Design review of the part built by this model. Coordinates are the model's own, in mm. A direction names the side the tool comes from. Give positions to 0.01 mm unless a question says otherwise; leave off trailing zeros. Loops run counter-clockwise (first coordinate to the right, second up) from the corner with the lowest first, then second, coordinate; pieces in that order, holes last. Notation, with made-up numbers: (72.5, -23) - (123.5, -23) arc R11 ccw to (123.5, -5) - close; hole circle Ø9 at (7, 20.25). An arc over 180 degrees is marked (long way). Put each result on its own line as item: value. Start each with the question number.
```python
from build123d import *

# Parameters (mm, degrees)
F0_R     = 6.35
F1_DEPTH = 5.08


with BuildPart() as f1:
    # F0 (on Top) → F1 (new body)
    with BuildSketch(Plane.XY):
        with BuildLine():
            Line((-4.392071, 35.177388), (-4.392071, 25.017388))
            ThreePointArc((-4.392071, 25.017388), (-7.849032, 24.156836), (-11.151592, 22.821087))
            Line((-11.151592, 22.821087), (-17.12349, 31.040699))
            ThreePointArc((-17.12349, 31.040699), (-21.638018, 29.782177), (-24.23001, 25.877511))
            Line((-24.23001, 25.877511), (-18.258112, 17.657898))
            ThreePointArc((-18.258112, 17.657898), (-20.549032, 14.929745), (-22.435726, 11.907905))
            Line((-22.435726, 11.907905), (-32.09846, 15.047518))
            ThreePointArc((-32.09846, 15.047518), (-35.011048, 11.375779), (-34.812909, 6.693303))
            Line((-34.812909, 6.693303), (-25.150175, 3.553691))
            ThreePointArc((-25.150175, 3.553691), (-25.4, 0), (-25.150175, -3.553691))
            Line((-25.150175, -3.553691), (-34.812909, -6.693303))
            ThreePointArc((-34.812909, -6.693303), (-35.011048, -11.375779), (-32.09846, -15.047518))
            Line((-32.09846, -15.047518), (-22.435726, -11.907905))
            ThreePointArc((-22.435726, -11.907905), (-20.549032, -14.929745), (-18.258112, -17.657898))
            Line((-18.258112, -17.657898), (-24.23001, -25.877511))
            ThreePointArc((-24.23001, -25.877511), (-21.638018, -29.782177), (-17.12349, -31.040699))
            Line((-17.12349, -31.040699), (-11.151592, -22.821087))
            ThreePointArc((-11.151592, -22.821087), (-7.849032, -24.156836), (-4.392071, -25.017388))
            Line((-4.392071, -25.017388), (-4.392071, -35.177388))
            ThreePointArc((-4.392071, -35.177388), (0, -36.812795), (4.392071, -35.177388))
            Line((4.392071, -35.177388), (4.392071, -25.017388))
            ThreePointArc((4.392071, -25.017388), (7.849032, -24.156836), (11.151592, -22.821087))
            Line((11.151592, -22.821087), (17.12349, -31.040699))
            ThreePointArc((17.12349, -31.040699), (21.638018, -29.782177), (24.23001, -25.877511))
            Line((24.23001, -25.877511), (18.258112, -17.657898))
            ThreePointArc((18.258112, -17.657898), (20.549032, -14.929745), (22.435726, -11.907905))
            Line((22.435726, -11.907905), (32.09846, -15.047518))
            ThreePointArc((32.09846, -15.047518), (35.011048, -11.375779), (34.812909, -6.693303))
            Line((34.812909, -6.693303), (25.150175, -3.553691))
            ThreePointArc((25.150175, -3.553691), (25.4, 0), (25.150175, 3.553691))
            Line((25.150175, 3.553691), (34.812909, 6.693303))
            ThreePointArc((34.812909, 6.693303), (35.011048, 11.375779), (32.09846, 15.047518))
            Line((32.09846, 15.047518), (22.435726, 11.907905))
            ThreePointArc((22.435726, 11.907905), (20.549032, 14.929745), (18.258112, 17.657898))
            Line((18.258112, 17.657898), (24.23001, 25.877511))
            ThreePointArc((24.23001, 25.877511), (21.638018, 29.782177), (17.12349, 31.040699))
            Line((17.12349, 31.040699), (11.151592, 22.821087))
            ThreePointArc((11.151592, 22.821087), (7.849032, 24.156836), (4.392071, 25.017388))
            Line((4.392071, 25.017388), (4.392071, 35.177388))
            ThreePointArc((4.392071, 35.177388), (0, 36.812795), (-4.392071, 35.177388))
        make_face()
        Circle(F0_R, mode=Mode.SUBTRACT)
    extrude(amount=F1_DEPTH)


solid = f1.part
```
Item 1: Consider section B-B (y = 0). State the section outline as (x, z) points, plus the area to 3 significant figures.
Item 2: Consider section A-A (x = 0). State the section outline as (y, z) points, plus the area to 3 significant figures.
Item 3: For L1, parallel to Y at x = -21, z = 0.3; L2, parallel to X at y = -27, z = 4.8; L3, parallel to X at y = 30.5, z = 3.8, list the stretches that pass through material, from the lowest coordinate up. Write a range as from..to.
Item 4: Consider section C-C (x = -21.5). State the section outline as (y, z) points.
Item 5: Mouldability with a two-part tool opening along Y and no side actions: class faces 1 (the flat face through (-14.096, 26.873, 2.504)), 2 (the flat face through (14.096, -26.873, 2.504)), 3 (the flat face through (-27.199, 13.456, 2.504)) as pulls with the +Y half, pulls with the -Y half, needs draft (parallel to the pull), parting line crosses it, or undercut.
Item 6: Consider section D-D (y = -29). State the section outline as (x, z) points, plus the area to 3 significant figures.
Item 7: Machinability: for faces 4 (the flat face through (21.2, 21.71, 2.5)), 5 (the cylindrical face through (-20.58, -14.89, 2.5)), 6 (the flat face through (4.392, -30, 3)), which of the approach directions +Z, -Z, +X, -X, +Y, -Y give a long, thin tool a straight path to every point of the face, cutting with its end or side? Answer none if there is none.
Item 8: For P1, Ø1, axis at y = 15, z = 2, coming from the +X side; P2, Ø3, axis at y = 24, z = 1, coming from the -X side; P3, Ø1, axis at x = 16.5, y = 9.5, coming from the -Z side; P4, Ø1.5, axis at y = -31, z = 3.5, coming from the +X side, all flat-tipped, find the tip position at first contact; note any pin that passes through.
Geometry says:
1. outline: (-25.4, 0) - (-6.35, 0) - (-6.35, 5.08) - (-25.4, 5.08) - close; (6.35, 0) - (25.4, 0) - (25.4, 5.08) - (6.35, 5.08) - close
1. area: 194 mm2
2. outline: (-36.81, 0) - (-6.35, 0) - (-6.35, 5.08) - (-36.81, 5.08) - close; (6.35, 0) - (36.81, 0) - (36.81, 5.08) - (6.35, 5.08) - close
2. area: 310 mm2
3. L1: y = -30.19..-21.43, -14.29..14.29, 21.43..30.19
3. L2: x = -23.86..-14.19, -4.39..4.39, 14.19..23.86
3. L3: x = -20.39..-16.73, -4.39..4.39, 16.73..20.39
4. outline: (-29.88, 0) - (-22.12, 0) - (-22.12, 5.08) - (-29.88, 5.08) - close; (-13.52, 0) - (13.52, 0) - (13.52, 5.08) - (-13.52, 5.08) - close; (22.12, 0) - (29.88, 0) - (29.88, 5.08) - (22.12, 5.08) - close
5. face 1: pulls with the +Y half
5. face 2: pulls with the -Y half
5. face 3: undercut
6. outline: (-22.54, 0) - (-15.64, 0) - (-15.64, 5.08) - (-22.54, 5.08) - close; (-4.39, 0) - (4.39, 0) - (4.39, 5.08) - (-4.39, 5.08) - close; (15.64, 0) - (22.54, 0) - (22.54, 5.08) - (15.64, 5.08) - close
6. area: 115 mm2
7. face 4: +Z, -Z, +X
7. face 5: +Z, -Z
7. face 6: +Z, -Z, -Y
8. P1: stops at x = 32.87
8. P2: stops at x = -23.96
8. P3: stops at z = 0
8. P4: stops at x = 20.9
